Read the model definition and answer for the solid it produces. Units are mm, in the model's axes. A direction names the side the tool comes from. Give positions to 0.01 mm unless a question says otherwise; leave off trailing zeros. Loops run counter-clockwise (first coordinate to the right, second up) from the corner with the lowest first, then second, coordinate; pieces in that order, holes last. Notation, with made-up numbers: (57, 49.25) - (61, 49.25) arc R19 cw to (61, 55.25) - close; hole circle Ø4 at (82, -16.5). An arc over 180 degrees is marked (long way). Write item = value, one per line.
```python
from build123d import *

# Parameters (mm, degrees)
F0_R     = 5
F1_DEPTH = 5.5
F2_W     = 5.25
F2_H     = 4
F3_DEPTH = 13
F4_R     = 0.75
F5_R     = 2.5
F6_DEPTH = 5


with BuildPart() as f1:
    # F0 (on Top) → F1 (new body)
    with BuildSketch(Plane.XY):
        Circle(F0_R)
    extrude(amount=F1_DEPTH)

    # F2 (on face) → F3 (join)
    with BuildSketch(Plane.XY.offset(5.5)):
        Rectangle(F2_W, F2_H)
    extrude(amount=F3_DEPTH)

    # F4
    f4_edges = [f1.edges().sort_by_distance(p)[0] for p in [
        (-2.625, -2, 12),
        (2.625, -2, 12),
        (2.625, 2, 12),
        (-2.625, 2, 12),
        (-2.625, 0, 5.5),
        (-2.625, 0, 18.5),
        (0, -2, 18.5),
        (2.625, 0, 18.5),
        (0, 2, 18.5),
        (0, -2, 5.5),
        (2.625, 0, 5.5),
        (0, 2, 5.5),
    ]]
    fillet(f4_edges, radius=F4_R)

    # F5 (on face) → F6 (cut)
    with BuildSketch(Plane(origin=(0, 0, 0), x_dir=(1, 0, 0), z_dir=(0, 0, -1))):
        Circle(F5_R)
    extrude(amount=-F6_DEPTH, mode=Mode.SUBTRACT)


solid = f1.part
```
1) A cutting plane is placed at B-B on z = 13. Determine the outline of the cut face in (x, y) (3 decimals), then the cut area to 3 significant figures.
Output:
outline = (-2.625, -1.25) arc R0.75 ccw to (-1.875, -2) - (1.875, -2) arc R0.75 ccw to (2.625, -1.25) - (2.625, 1.25) arc R0.75 ccw to (1.875, 2) - (-1.875, 2) arc R0.75 ccw to (-2.625, 1.25) - close
area = 20.5 mm²
2) Each of these flat-tipped pins is pushed along its axis until it touches: P1, Ø4, axis at y = 2.5, z = 4.5, coming from the -X side; P2, Ø1, axis at y = -1.5, z = 3, coming from the +X side; P3, Ø2, axis at y = 0, z = 14, coming from the +X side (3 decimals). Where does it stop, or does it pass through?
Output:
P1 = -4.97
P2 = 4.9
P3 = 2.625
3) Find the intervals of material crossed by probe 1 along Y at (x, z) = (0, 1.45); probe 2 along Y at (x, z) = (0, 15.25); probe 3 along Z at (x, y) = (0.25, -4.25), in increasing order.
Output:
probe_1 = -5 to -2.5, 2.5 to 5
probe_2 = -2 to 2
probe_3 = 0 to 5.5
4) A tool of negligible diameter and unlimited length cuts with its end or side. For faces 1 (the face through (-2.625, 0, 12)), 2 (the face through (0, 0, 18.5)), 3 (the face through (0, -2, 12)), 4 (the face through (2.625, 0, 12)), 5 (the face through (0, 2, 12)), from which of +Z, -Z, +X, -X, +Y, -Y can it reach the whole face along a straight path? Write none if from no direction.
Output:
face_1 = +Z, -X, +Y, -Y
face_2 = +Z, +X, -X, +Y, -Y
face_3 = +Z, +X, -X, -Y
face_4 = +Z, +X, +Y, -Y
face_5 = +Z, +X, -X, +Y
5) A cutting plane is placed at D-D on x = 4. Determine the outline of the cut face in (y, z), then the cut area to 3 significant figures.
Output:
outline = (-3, 0) - (3, 0) - (3, 5.5) - (-3, 5.5) - close
area = 33.0 mm²
6) A cutting plane is placed at A-A on x = 0. Determine the outline of the cut face in (y, z), then the cut area to 3 significant figures.
Output:
outline = (-5, 0) - (-2.5, 0) - (-2.5, 5) - (2.5, 5) - (2.5, 0) - (5, 0) - (5, 5.5) - (2.75, 5.5) arc R0.75 cw to (2, 6.25) - (2, 17.75) arc R0.75 ccw to (1.25, 18.5) - (-1.25, 18.5) arc R0.75 ccw to (-2, 17.75) - (-2, 6.25) arc R0.75 cw to (-2.75, 5.5) - (-5, 5.5) - close
area = 82.0 mm²
7) The mould has two halves that part along X. Classify faces 6 (the face through (0, -3, 5.5)), 7 (the face through (-1.08, -4.88, 2.71)), 8 (the face through (-0.54, 2.44, 2.46)), 9 (the face through (0, 0, 5)): pulls with the +X half, pulls with the -X half, needs draft (parallel to the pull), parting line crosses it, or undercut.
Output:
face_6 = needs draft
face_7 = parting line crosses it
face_8 = undercut
face_9 = undercut
8) A cutting plane is placed at C-C on y = 0. Determine the outline of the cut face in (x, z) (3 decimals).
Output:
outline = (-5, 0) - (-2.5, 0) - (-2.5, 5) - (2.5, 5) - (2.5, 0) - (5, 0) - (5, 5.5) - (3.375, 5.5) arc R0.75 cw to (2.625, 6.25) - (2.625, 17.75) arc R0.75 ccw to (1.875, 18.5) - (-1.875, 18.5) arc R0.75 ccw to (-2.625, 17.75) - (-2.625, 6.25) arc R0.75 cw to (-3.375, 5.5) - (-5, 5.5) - close
